Design review of the part built by this model. Coordinates are the model's own, in mm. Face numbers are marked on the shaded views. A direction names the side the tool comes from. Give positions to 0.01 mm unless a question says otherwise; leave off trailing zeros. Order: outer loops, then holes, each group sorted by start corner. A loop starts at its lowest first (then second) coordinate and runs counter-clockwise, first axis right, second up. Notation, with made-up numbers: (53, -33) - (96, -33) arc R29 cw to (96, -4) - close; hole circle Ø2 at (20, 44.5). An arc over 180 degrees is marked (long way). Write each question's results on one line, items separated by ' | '. Start each with the question number.
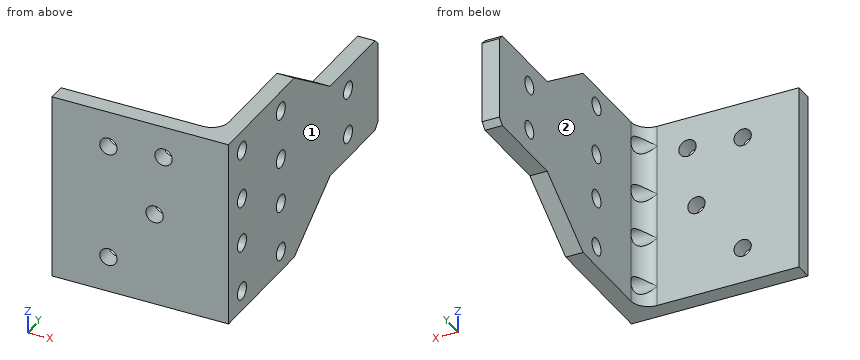
Autodesk Inventor part; units mm, degrees
ref_plane "YZ Plane" through (0, 0, 0) normal (1, 0, 0) x (0, 1, 0)
ref_plane "XZ Plane" through (0, 0, 0) normal (0, 1, 0) x (-1, 0, 0)
ref_plane "XY Plane" through (0, 0, 0) normal (0, 0, 1) x (1, 0, 0)
sketch "Szkic1" plane through (0, 0, 0) normal (0, 0, 1) x (1, 0, 0)
  line L0 (-15.1556, -3.6171) -> (-15.1556, -6.6171)
  line L1 (-15.1556, -6.6171) -> (15.3944, -6.6171)
  line L2 (15.3944, -6.6171) -> (15.3944, 15.3829)
  line L3 (15.3944, 15.3829) -> (12.3944, 15.3829)
  line L4 (12.3944, 15.3829) -> (12.3944, -3.6171)
  line L5 (12.3944, -3.6171) -> (-15.1556, -3.6171)
  point P0 (0, 0)
  dimension "d0" = 3
  dimension "d1" = 30.55
  dimension "d2" = 22
  dimension "d3" = 3
extrude "Wyciągnięcie proste1" add sketch "Szkic1" along normal blind 32.4
fillet "Zaokrąglenie1" radius 3 1 edges at (12.3944, -3.6171, 16.2)
sketch "Szkic3" plane through (15.3944, -6.6171, 32.4) normal (1, 0, 0) x (0, 0, -1)
  line L0 (32.4, 22) -> (0, 22)
  line L1 (0, 0) -> (0, 22)
  line L2 (32.4, 0) -> (0, 0)
  line L3 (32.4, 0) -> (32.4, 22)
  line L4 (32.4, 22) -> (0, 22)
  line L5 (24.3, 22) -> (8.1, 22)
  line L6 (8.1, 22) -> (8.1, 50)
  line L7 (8.1, 50) -> (24.3, 50)
  line L8 (24.3, 50) -> (24.3, 22)
  point P0 (32.4, 6.6171)
  dimension "d48" = 16.2
  dimension "d49" = 28
  dimension "d50" = 32.4
  dimension "d51" = 8.1
extrude "Wyciągnięcie proste3" add sketch "Szkic3" against normal blind 3 contours L0 L6 L7 L8
sketch "Szkic4" plane through (-15.1556, -6.6171, 0) normal (0, -1, 0) x (1, 0, 0)
  line L0 (0, 0) -> (30.55, 0)
  line L1 (30.55, 0) -> (30.55, 32.4)
  line L2 (0, 32.4) -> (30.55, 32.4)
  line L3 (0, 0) -> (0, 32.4)
  point P0 (15.1556, 0)
  point P1 (9.75, 26.2)
  point P2 (9.75, 6.2)
  point P3 (17.75, 16.2)
  dimension "d37" = 9.75
  dimension "d38" = 9.75
  dimension "d39" = 6.2
  dimension "d40" = 6.2
  dimension "d69" = 32.4
  dimension "d70" = 16.2
  dimension "d71" = 17.75
hole "Otwór2" at (-5.4056, -6.6171, 26.2) at (-5.4056, -6.6171, 6.2) at (2.5944, -6.6171, 16.2) direction (0, 1, 0) diameter 3 end through all
sketch "Szkic5" plane through (15.3944, -6.6171, 0) normal (1, 0, 0) x (0, 0, -1)
  line L0 (0, 0) -> (0, 22)
  line L1 (0, 22) -> (-8.1, 22)
  line L2 (-8.1, 22) -> (-8.1, 50)
  line L3 (-8.1, 50) -> (-24.3, 50)
  line L4 (-24.3, 50) -> (-24.3, 22)
  line L5 (-24.3, 22) -> (-32.4, 22)
  line L6 (-32.4, 0) -> (-32.4, 22)
  line L7 (0, 0) -> (-32.4, 0)
  point P0 (0, 6.6171)
  point P1 (-12.3, 40)
  point P2 (-20.3, 40)
  dimension "d52" = 10
  dimension "d53" = 10
  dimension "d54" = 4
  dimension "d55" = 4.2
hole "Otwór3" at (15.3944, 33.3829, 12.3) at (15.3944, 33.3829, 20.3) direction (-1, 0, 0) diameter 3 end through all
chamfer "Faza2" distance 1 angle 45 2 edges at (13.8944, 43.3829, 24.3) (13.8944, 43.3829, 8.1)
chamfer "Faza4" distance 8.1 distance2 12 1 edges at (13.8944, 15.3829, 24.3) measured on face at (14.3944, 15.3829, 27)
chamfer "Faza5" distance 8.1 distance2 12 1 edges at (13.8944, 15.3829, 8.1) measured on face at (14.3944, 15.3829, 2.7)
sketch "Szkic6" plane through (15.3944, -6.6171, 32.4) normal (1, 0, 0) x (0, 0, -1)
  circle A0 centre (20.1, 40) radius 1.5
  circle A1 centre (12.1, 40) radius 1.5
  line L0 (23.3, 50) -> (24.3, 49)
  line L1 (23.3, 50) -> (9.1, 50)
  line L2 (8.1, 49) -> (9.1, 50)
  line L3 (8.1, 49) -> (8.1, 34)
  line L4 (0, 22) -> (8.1, 34)
  line L5 (0, 0) -> (0, 22)
  line L6 (32.4, 0) -> (0, 0)
  line L7 (32.4, 0) -> (32.4, 22)
  line L8 (24.3, 34) -> (32.4, 22)
  line L9 (24.3, 34) -> (24.3, 49)
  point P0 (32.4, 6.6171)
  point P1 (3.5, 17.5)
  point P2 (3.5, 4.5)
  point P3 (28.9, 17.5)
  point P4 (28.9, 4.5)
  point P5 (35.2902, 42.5614)
  point P6 (12.2, 17.5)
  point P7 (12.2, 4.5)
  point P8 (20.2, 17.5)
  point P9 (20.2, 4.5)
  dimension "d79" = 3.5
  dimension "d80" = 3.5
  dimension "d81" = 3.5
  dimension "d82" = 3.5
  dimension "d83" = 4.5
  dimension "d84" = 4.5
  dimension "d85" = 13
  dimension "d86" = 13
  dimension "d87" = 8.7
  dimension "d88" = 8.7
  dimension "d89" = 8.7
  dimension "d90" = 8.7
hole "Otwór4" at (15.3944, 10.8829, 28.9) at (15.3944, -2.1171, 28.9) at (15.3944, 10.8829, 3.5) at (15.3944, -2.1171, 3.5) at (15.3944, 35.9442, -2.8902) at (15.3944, 10.8829, 20.2) at (15.3944, -2.1171, 20.2) at (15.3944, 10.8829, 12.2) at (15.3944, -2.1171, 12.2) direction (-1, 0, 0) diameter 3 end through all
sketch "Szkic7" plane through (-15.1556, -6.6171, 0) normal (0, -1, 0) x (1, 0, 0)
  circle A0 centre (9.75, 6.2) radius 1.5
  circle A1 centre (9.75, 26.2) radius 1.5
  circle A2 centre (17.75, 16.2) radius 1.5
  line L0 (0, 0) -> (30.55, 0)
  line L1 (30.55, 0) -> (30.55, 32.4)
  line L2 (0, 32.4) -> (30.55, 32.4)
  line L3 (0, 0) -> (0, 32.4)
  point P0 (15.1556, 0)
  point P1 (19.3, 26.96)
  dimension "d98" = 5.44
  dimension "d99" = 19.3
hole "Otwór5" at (4.1444, -6.6171, 26.96) direction (0, 1, 0) diameter 3 depth 8 tip angle 118
equation "\"d51\" = -0.5 * d48 + 0.5 * d50"
properties part number "CNCM_X_Axiss_Carriage_Belt_and_Cable_Chain_Mount"
Q1. Add section A-A (z = 6.5). Give the boundary of the cut face in (x, y).
Q2. Machinability: for the marked faces 1 and 2, which of the approach directions +Z, -Z, +X, -X, +Y, -Y give a long, thin tool a straight path to every point of the face, cutting with its end or side? Answer none if there is none.
Q3. Insertion check: pin 1 Ø1 at (x, z) = (7.5, 6.5) entering from +Y; pin 2 Ø2.5 at (x, z) = (-5.41, 6.2) entering from -Y; pin 3 Ø4 at (y, z) = (10.88, 28.9) entering from +X; pin 4 Ø1.5 at (y, z) = (6.5, 11) entering from -X. Each pin has a flat end and moves straight along its axis. Give the tip position at first contact, or say it passes through.
Q4. Add section C-C (y = 37). Give the boundary of the cut face in (x, z).
Q5. Add section D-D (x = 8). Give the boundary of the cut face in (y, z).
Q6. For line 1 (Y direction, x = 14.45, z = 12.3); line 2 (X direction, y = -5, z = 6); line 3 (X direction, y = 19.5, z = 21.5), list the stretches that pass through material, from the lowest coordinate up. Write a range as [from, to].
Q7. Add section B-B (z = 11.5). Give the boundary of the cut face in (x, y), plus the area to 3 significant figures.
Verdict:
1) outline: (-15.16, -6.62) - (-6.88, -6.62) - (-6.88, -3.62) - (-15.16, -3.62) - close; (-3.94, -6.62) - (15.39, -6.62) - (15.39, 25.01) - (12.39, 25.01) - (12.39, -0.62) arc R3 cw to (9.39, -3.62) - (-3.94, -3.62) - close
2) face 1: +Z, -Z, +X, +Y, -Y | face 2: +Z, -Z, -X, +Y
3) pin 1: stops at y = -3.62 | pin 2: passes through | pin 3: stops at x = 15.39 | pin 4: stops at x = 12.39
4) outline: (12.39, 8.1) - (15.39, 8.1) - (15.39, 24.3) - (12.39, 24.3) - close
5) outline: (-6.62, 0) - (-3.62, 0) - (-3.62, 32.4) - (-6.62, 32.4) - close
6) line 1: y = [-6.62, -3.61], [-0.62, 9.39], [12.38, 31.88], [34.88, 43.38] | line 2: x = [-15.16, -6.89], [-3.92, 15.39] | line 3: x = [12.39, 15.39]
7) outline: (-15.16, -6.62) - (15.39, -6.62) - (15.39, -3.44) - (10.4, -3.44) arc R3 cw to (9.39, -3.62) - (-15.16, -3.62) - close; (12.39, -0.79) - (15.39, -0.79) - (15.39, 9.56) - (12.39, 9.56) - (12.39, -0.62) arc R3 cw to start; (12.39, 12.21) - (15.39, 12.21) - (15.39, 32.11) - (12.39, 32.11) - close; (12.39, 34.65) - (15.39, 34.65) - (15.39, 43.38) - (12.39, 43.38) - close | area: 210 mm2
